Can you work these out from the model? Positions are in its coordinate system, mm. A direction names the side the tool comes from. Give positions to 0.01 mm unless a question says otherwise; leave off trailing zeros. Write each loop counter-clockwise with the first axis right and the second up, starting at its lowest first coordinate (ties: lowest second). Pieces come first, ordered by that corner, then holes. Notation, with made-up numbers: M 8,74 L 56,74 A22 ccw 56,88 Z; hole C 28,44.25 d7. An arc over 180 degrees is marked long. Write each question's results on one line, items separated by ' | '.
from build123d import *

# Parameters (mm, degrees)
F0_W     = 266.7
F0_H     = 127
F1_DEPTH = 31.75
F3_DEPTH = 209.55
F4_D     = 5


with BuildPart() as f1:
    # F0 (on Top) → F1 (new body)
    with BuildSketch(Plane.XY):
        Rectangle(F0_W, F0_H)
    extrude(amount=F1_DEPTH)

    # F2 (on face) → F3 (join)
    with BuildSketch(Plane.XY.offset(31.75)):
        with BuildLine():
            Line((-42.1211348375, 63.5), (42.1211348375, 63.5))
            ThreePointArc((42.1211348375, 63.5), (0, 76.2), (-42.1211348375, 63.5))
        make_face()
        with BuildLine():
            ThreePointArc((42.1211348375, -63.5), (67.1419037361, -36.0333840028), (76.2, 0))
            ThreePointArc((76.2, 0), (67.1419037361, 36.0333840028), (42.1211348375, 63.5))
            Line((42.1211348375, 63.5), (-42.1211348375, 63.5))
            ThreePointArc((-42.1211348375, 63.5), (-76.2, 0), (-42.1211348375, -63.5))
            Line((-42.1211348375, -63.5), (42.1211348375, -63.5))
        make_face()
        with BuildLine():
            ThreePointArc((-42.1211348375, -63.5), (0, -76.2), (42.1211348375, -63.5))
            Line((42.1211348375, -63.5), (-42.1211348375, -63.5))
        make_face()
    extrude(amount=F3_DEPTH)

    # F4 (through all)
    with Locations(Plane(origin=(0, 0, 0), x_dir=(1, 0, 0), z_dir=(0, 0, -1))):
        with Locations((88.9, -63.5), (88.9, 63.5), (0, 63.5), (0, -63.5), (0, 0)):
            Hole(F4_D / 2)


solid = f1.part
Item 1: I'm going to push flat-ended pins straight in: pin 1 (1.5 mm diameter, centred on x = 14.5, z = 182.5, fed in from -Y); pin 2 (3 mm diameter, centred on x = -44, z = 179, fed in from -Y); pin 3 (1.5 mm diameter, centred on y = -2, z = 94, fed in from +X). Where does each tip first touch, or does it pass through?
Geometry says:
pin 1: stops at y = -74.95 | pin 2: stops at y = -63.25 | pin 3: stops at x = 76.19
Item 2: If I drill on line 1 (Y direction, x = 0, z = 142); line 2 (X direction, y = -63.5, z = 168); line 3 (Z direction, x = -77.5, y = -50), over which ranges is the centre line in solid material (lowest first)? Write a range as from..to.
Geometry says:
line 1: y = -76.2..-66, -61..-2.5, 2.5..61, 66..76.2 | line 2: x = -42.12..-2.5, 2.5..42.12 | line 3: z = 0..31.75
Item 3: For faces 1 (the face through (44, 63.5, 16)), 2 (the face through (44, -63.5, 16)), 3 (the face through (5.21, -76.02, 135.06)), which set-ups out of +Z, -Z, +X, -X, +Y, -Y let a thin tool reach every point of the face, with its end or its side?
Geometry says:
face 1: -Z, +X, -X, +Y | face 2: -Z, +X, -X, -Y | face 3: +Z
Item 4: I want a section at C-C, the plane y = -42.5. Please give me the cut outline in (x, z).
Geometry says:
outline: M -133.35,0 L 133.35,0 L 133.35,31.75 L 63.25,31.75 L 63.25,241.3 L -63.25,241.3 L -63.25,31.75 L -133.35,31.75 Z
Item 5: I want a section at A-A, the plane x = -20.5. Please give me the cut outline in (y, z), and give its area (3 significant figures).
Geometry says:
outline: M -73.39,31.75 L -63.5,31.75 L -63.5,0 L 63.5,0 L 63.5,31.75 L 73.39,31.75 L 73.39,241.3 L -73.39,241.3 Z | area: 34,800 mm2
Item 6: I want a section at B-B, the plane z = 150. Please give me the cut outline in (x, y).
Geometry says:
outline: C 0,0 d152.4; hole C 0,-63.5 d5; hole C 0,0 d5; hole C 0,63.5 d5
Item 7: I want a section at D-D, the plane x = -95. Please give me the cut outline in (y, z).
Geometry says:
outline: M -63.5,0 L 63.5,0 L 63.5,31.75 L -63.5,31.75 Z
